Geometry check sheet. Reference: the model listing, model coordinates, mm. Face numbers are marked on the shaded views. A direction names the side the tool comes from. Round coordinates to 2 decimals unless told otherwise and drop trailing zeros. Order: outer loops, then holes, each group sorted by start corner. A loop starts at its lowest first (then second) coordinate and runs counter-clockwise, first axis right, second up. Notation, with made-up numbers: (72.25, 44.25) -> (129.25, 44.25) arc R6 cw to (129.25, 48.25) -> close; hole circle Ø11 at (75, 35). An arc over 180 degrees is marked (long way). Use a Markdown table: item, result. Add a question column.
Item 1: Sectioned sample at B-B, the plane z = -13. Record the cut outline in (x, y).
Item 2: Gauge pin test, flat ends, axial feed: pin 1 Ø5 at (y, z) = (6.5, -76.5) entering from +X; pin 2 Ø6 at (x, z) = (28, -147) entering from -Y; pin 3 Ø1.5 at (y, z) = (32, -74.5) entering from -X; pin 4 Ø12 at (y, z) = (22, -41) entering from +X. Record the tip position at first contact, or that the pin passes through.
Item 3: Material ranges on probe 1 along X at (y, z) = (7.75, -115); probe 2 along X at (y, z) = (49.5, -15); probe 3 along Z at (x, y) = (55, 47), recorded low to high. Write a range as [from, to].
Item 4: Sectioned sample at A-A, the plane x = 48. Record the cut outline in (y, z), and give its area (3 significant figures).
Item 5: Mould release check, pull along Z, two halves, no side actions. Record for the marked faces 1 and 2: pulls with the +Z half, pulls with the -Z half, needs draft (parallel to the pull), parting line crosses it, or undercut.
Item 6: Set-up check for the marked faces 3, 4 and 5: record each of +Z, -Z, +X, -X, +Y, -Y from which the full face is reachable in a straight line by a thin tool's end or side.
Item 7: Sectioned sample at D-D, the plane z = -50. Record the cut outline in (x, y) (3 decimals).
Item 8: Sectioned sample at C-C, the plane y = 43.5. Record the cut outline in (x, z), and give its area (3 significant figures).
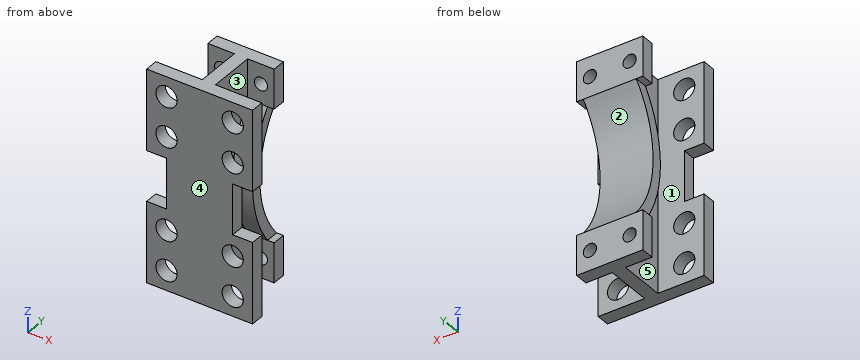
from build123d import *

# Parameters (mm, degrees)
SKETCH1_R           = 8
BOSS_EXTRUDE1_DEPTH = 10
BOSS_EXTRUDE2_DEPTH = 5
SKETCH7_W           = 50
SKETCH7_H           = 30
SKETCH7_R           = 5
BOSS_EXTRUDE3_DEPTH = 10
BOSS_EXTRUDE5_DEPTH = 20
CUT_EXTRUDE1_DEPTH  = 20


with BuildPart() as part:
    # Sketch1 → Boss-Extrude1 (new body)
    with BuildSketch(Plane(origin=(0, 0, 0), x_dir=(1, 0, 0), z_dir=(0, 1, 0))):
        Polygon((80, 160), (0, 160), (0, 99), (15, 99), (15, 61), (0, 61), (0, 0), (80, 0), (80, 61), (65, 61), (65, 99), (80, 99), align=None)
        with Locations((15, 15)):
            Circle(SKETCH1_R, mode=Mode.SUBTRACT)
        with Locations((15, 45)):
            Circle(SKETCH1_R, mode=Mode.SUBTRACT)
        with Locations((65, 15)):
            Circle(SKETCH1_R, mode=Mode.SUBTRACT)
        with Locations((65, 45)):
            Circle(SKETCH1_R, mode=Mode.SUBTRACT)
        with Locations((15, 115)):
            Circle(SKETCH1_R, mode=Mode.SUBTRACT)
        with Locations((15, 145)):
            Circle(SKETCH1_R, mode=Mode.SUBTRACT)
        with Locations((65, 115)):
            Circle(SKETCH1_R, mode=Mode.SUBTRACT)
        with Locations((65, 145)):
            Circle(SKETCH1_R, mode=Mode.SUBTRACT)
    extrude(amount=BOSS_EXTRUDE1_DEPTH)

    # Sketch2 → Boss-Extrude2 (add, symmetric)
    with BuildSketch(Plane(origin=(40, 0, 0), x_dir=(0, 0, -1), z_dir=(1, 0, 0))):
        Polygon((160, 10), (99, 10), (61, 10), (0, 10), (0, 45), (160, 45), align=None)
    extrude(amount=BOSS_EXTRUDE2_DEPTH, both=True)

    # Sketch7 → Boss-Extrude3 (add)
    with BuildSketch(Plane(origin=(0, 45, 0), x_dir=(-1, 0, 0), z_dir=(0, -1, 0))):
        with Locations((-40, 15)):
            Rectangle(SKETCH7_W, SKETCH7_H)
        with Locations((-55, 15)):
            Circle(SKETCH7_R, mode=Mode.SUBTRACT)
        with Locations((-25, 15)):
            Circle(SKETCH7_R, mode=Mode.SUBTRACT)
        with Locations((-40, 145)):
            Rectangle(SKETCH7_W, SKETCH7_H)
        with Locations((-25, 145)):
            Circle(SKETCH7_R, mode=Mode.SUBTRACT)
        with Locations((-55, 145)):
            Circle(SKETCH7_R, mode=Mode.SUBTRACT)
    extrude(amount=-BOSS_EXTRUDE3_DEPTH)

    # Sketch12 → Boss-Extrude5 (add, symmetric)
    with BuildSketch(Plane(origin=(40, 0, 0), x_dir=(0, 0, -1), z_dir=(1, 0, 0))):
        with BuildLine():
            ThreePointArc((30, 45), (80, 28.829043194), (130, 45))
            Line((130, 45), (114.867292292, 45))
            ThreePointArc((114.867292292, 45), (80, 36.713596412), (45.132707708, 45))
            Line((45.132707708, 45), (30, 45))
        make_face()
        with BuildLine():
            Line((30, 55), (30, 45))
            Line((30, 45), (45.132707708, 45))
            ThreePointArc((45.132707708, 45), (37.272791745, 49.555761041), (30, 55))
        make_face()
        with BuildLine():
            Line((114.867292292, 45), (130, 45))
            Line((130, 45), (130, 55))
            ThreePointArc((130, 55), (122.727208255, 49.555761041), (114.867292292, 45))
        make_face()
    extrude(amount=BOSS_EXTRUDE5_DEPTH, both=True)

    # Sketch10 → Cut-Extrude1 (cut, symmetric)
    with BuildSketch(Plane(origin=(45, 0, 0), x_dir=(0, 0, -1), z_dir=(1, 0, 0))):
        with BuildLine():
            Line((114.867292292, 45), (45.132707708, 45))
            ThreePointArc((45.132707708, 45), (80, 36.713596412), (114.867292292, 45))
        make_face()
    extrude(amount=CUT_EXTRUDE1_DEPTH, both=True, mode=Mode.SUBTRACT)


solid = part.part
Found:
| question | item | result |
|---|---|---|
| 1 | outline | (0, 0) -> (7.25, 0) -> (7.25, 10) -> (0, 10) -> close; (15, 45) -> (20.42, 45) -> (20.42, 55) -> (15, 55) -> close; (22.75, 0) -> (57.25, 0) -> (57.25, 10) -> (45, 10) -> (45, 45) -> (50.42, 45) -> (50.42, 55) -> (29.58, 55) -> (29.58, 45) -> (35, 45) -> (35, 10) -> (22.75, 10) -> close; (59.58, 45) -> (65, 45) -> (65, 55) -> (59.58, 55) -> close; (72.75, 0) -> (80, 0) -> (80, 10) -> (72.75, 10) -> close |
| 2 | pin 1 | stops at x = 65 |
| 2 | pin 2 | stops at y = 0 |
| 2 | pin 3 | stops at x = 20 |
| 2 | pin 4 | stops at x = 45 |
| 3 | probe 1 | x = [0, 7], [23, 57], [73, 80] |
| 3 | probe 2 | x = [15, 20], [30, 50], [60, 65] |
| 3 | probe 3 | z = [-160, -150], [-140, -118.58], [-41.42, -20], [-10, 0] |
| 4 | outline | (0, -160) -> (10, -160) -> (10, 0) -> (0, 0) -> close; (45, -160) -> (55, -160) -> (55, -130) arc R77.5 cw to (55, -30) -> (55, 0) -> (45, 0) -> (45, -30) arc R85.38 ccw to (45, -130) -> close |
| 4 | area | 3,050 mm2 |
| 5 | face 1 | needs draft |
| 5 | face 2 | undercut |
| 6 | face 3 | +X |
| 6 | face 4 | +Z, -Z, +X, -X, -Y |
| 6 | face 5 | -X |
| 7 | outline | (0, 0) -> (8.755, 0) -> (8.755, 10) -> (0, 10) -> close; (20, 34.273) -> (35, 34.273) -> (35, 10) -> (21.245, 10) -> (21.245, 0) -> (58.755, 0) -> (58.755, 10) -> (45, 10) -> (45, 34.273) -> (60, 34.273) -> (60, 42.756) -> (20, 42.756) -> close; (71.245, 0) -> (80, 0) -> (80, 10) -> (71.245, 10) -> close |
| 8 | outline | (20, -127.86) -> (35, -127.86) -> (35, -160) -> (45, -160) -> (45, -127.86) -> (60, -127.86) -> (60, -111.71) -> (20, -111.71) -> close; (20, -48.29) -> (60, -48.29) -> (60, -32.14) -> (45, -32.14) -> (45, 0) -> (35, 0) -> (35, -32.14) -> (20, -32.14) -> close |
| 8 | area | 1,930 mm2 |
